Source: CAD feature listing. Evaluate the final solid. Frame: model axes, mm. Face numbers are marked on the shaded views. A direction names the side the tool comes from. Give positions to 0.01 mm unless a question says otherwise; leave off trailing zeros. Order: outer loops, then holes, each group sorted by start corner. A loop starts at its lowest first (then second) coordinate and runs counter-clockwise, first axis right, second up.
from build123d import *

# Parameters (mm, degrees)
MAIN_BODY_DEPTH                 = 75
SKETCH6_W                       = 38
SKETCH6_H                       = 25
BASE_FIT_PLATE_DEPTH            = 4
SKETCH3_W                       = 3.2102875
SKETCH3_H                       = 3
FRONT_SCREW_HOLES_SUPPORT_DEPTH = 6
FRONT_SCREW_HOLES_REACH         = 79.891
SKETCH4_R                       = 1.05
SKETCH7_W                       = 29
SKETCH7_H                       = 20
SKETCH7_R                       = 8
BUTTON_HOLE_DEPTH               = 2
SKETCH8_W                       = 22
SKETCH8_H                       = 25
SKETCH8_W_2                     = 13.3
SKETCH8_H_2                     = 21.3
SWITCH_HOLE_DEPTH               = 8
SKETCH9_R                       = 1.1
BASE_SCREW_HOLES_DEPTH          = 81.051545894


with BuildPart() as part:
    # Sketch1 → Main Body (new body)
    with BuildSketch(Plane(origin=(0, 0, 0), x_dir=(1, 0, 0), z_dir=(0, 1, 0))):
        with BuildLine():
            Line((0, 4.2897125), (-3.715, 2.14485625))
            Line((-3.715, 2.14485625), (-3.715, -2.14485625))
            Line((-3.715, -2.14485625), (0, -4.2897125))
            Line((0, -4.2897125), (0, -7.5))
            ThreePointArc((0, -7.5), (-7.5, 0), (0, 7.5))
            Line((0, 7.5), (0, 4.2897125))
        make_face()
    extrude(amount=MAIN_BODY_DEPTH)

    # Sketch6 → Base Fit Plate (add)
    with BuildSketch(Plane(origin=(-5, 0, 0), x_dir=(0, 0, -1), z_dir=(1, 0, 0))):
        with Locations((0, -2.5)):
            Rectangle(SKETCH6_W, SKETCH6_H)
    extrude(amount=-BASE_FIT_PLATE_DEPTH)

    # Sketch3 → Front Screw Holes Support (add)
    with BuildSketch(Plane(origin=(0, 0, 0), x_dir=(0, 0, -1), z_dir=(1, 0, 0))):
        with Locations((-5.89485625, 1.5)):
            Rectangle(SKETCH3_W, SKETCH3_H)
        with Locations((-5.89485625, 73.5)):
            Rectangle(SKETCH3_W, SKETCH3_H)
    front_screw_holes_support = extrude(amount=-FRONT_SCREW_HOLES_SUPPORT_DEPTH)

    # Sketch4 → Front Screw Holes (cut, up to next)
    with BuildSketch(Plane(origin=(0, 0, 0), x_dir=(0, 0, -1), z_dir=(1, 0, 0)), mode=Mode.PRIVATE) as front_screw_holes_sk1:
        with Locations((-5.89485625, 73.5)):
            Circle(SKETCH4_R)
    front_screw_holes_tool1 = extrude(front_screw_holes_sk1.sketch, amount=-FRONT_SCREW_HOLES_REACH, mode=Mode.PRIVATE) & part.part
    # Sketch4 → Front Screw Holes (cut, up to next)
    with BuildSketch(Plane(origin=(0, 0, 0), x_dir=(0, 0, -1), z_dir=(1, 0, 0)), mode=Mode.PRIVATE) as front_screw_holes_sk2:
        with Locations((-5.89485625, 1.5)):
            Circle(SKETCH4_R)
    front_screw_holes_tool2 = extrude(front_screw_holes_sk2.sketch, amount=-FRONT_SCREW_HOLES_REACH, mode=Mode.PRIVATE) & part.part
    front_screw_holes_1 = front_screw_holes_tool1.solids().sort_by_distance((0, 73.5, 5.894856))[0]
    add(front_screw_holes_1, mode=Mode.SUBTRACT)
    front_screw_holes_2 = front_screw_holes_tool2.solids().sort_by_distance((0, 1.5, 5.894856))[0]
    add(front_screw_holes_2, mode=Mode.SUBTRACT)
    front_screw_holes = front_screw_holes_1 + front_screw_holes_2  # Front Screw Holes as one shape, for the pattern or mirror that repeats it

    # Back Screw Holes and Support: Front Screw Holes Support, Front Screw Holes across plane
    add(front_screw_holes_support.mirror(Plane.XY))
    add(front_screw_holes.mirror(Plane.XY), mode=Mode.SUBTRACT)

    # Sketch7 → Button Hole (add)
    with BuildSketch(Plane(origin=(-5, 0, 0), x_dir=(0, 0, -1), z_dir=(1, 0, 0))):
        with Locations((12, 20)):
            Rectangle(SKETCH7_W, SKETCH7_H)
        with Locations((16, 20)):
            Circle(SKETCH7_R, mode=Mode.SUBTRACT)
    extrude(amount=-BUTTON_HOLE_DEPTH)

    # Sketch8 → Switch Hole (add)
    with BuildSketch(Plane(origin=(-5, 0, 0), x_dir=(0, 0, -1), z_dir=(1, 0, 0))):
        with Locations((15, 42)):
            Rectangle(SKETCH8_W, SKETCH8_H)
        with Locations((15, 42)):
            Rectangle(SKETCH8_W_2, SKETCH8_H_2, mode=Mode.SUBTRACT)
    extrude(amount=-SWITCH_HOLE_DEPTH)

    # Sketch9 → Base Screw Holes (cut, through all)
    with BuildSketch(Plane.ZY.offset(9)):
        with Locations((-13, 3)):
            Circle(SKETCH9_R)
        with Locations((13, 3)):
            Circle(SKETCH9_R)
    extrude(amount=-BASE_SCREW_HOLES_DEPTH, mode=Mode.SUBTRACT)


solid = part.part
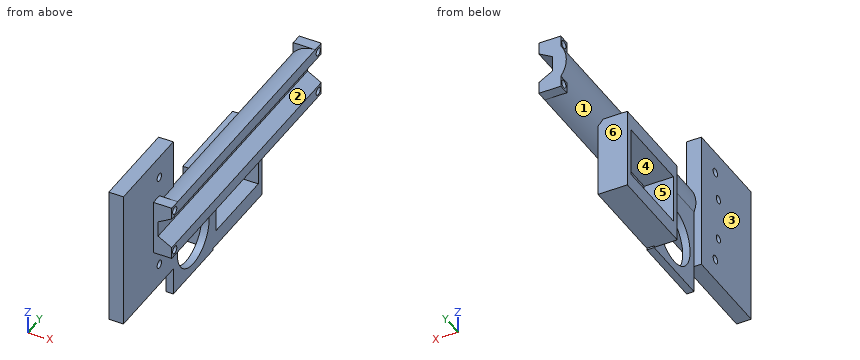
(1) Draft query along Z for the marked faces 5 and 6. Return one class per face: +Z half, -Z half, draft (parallel to the pull), parting line (faces both ways), or undercut.
(2) Section C-C, the plane x = -2.5. Return loops of the section in (y, z), plus the area to 3 significant figures.
(3) Access query for the marked faces 1, 2, 3 and 4. Directions: +Z, -Z, +X, -X, +Y, -Y. A direction counts if a zero-diameter tool reaches every point of the face in a straight line with its end or side. Return the directions, or none.
(4) Pin query (flat end, axial travel): pin 1 Ø4.5 at (x, y) = (-8, 1) entering from -Z; pin 2 Ø1.5 at (y, z) = (74, -5.5) entering from -X; pin 3 Ø4 at (x, z) = (-10, -13.5) entering from +Y. Return the tip coordinate at first contact, or that it passes through.
(5) Section B-B, the plane y = 20. Return loops of the section in (x, z) (3 decimals), plus the area to 3 significant figures.
(6) Line query: line 1 along Y through (x, z) = (-11, -11); line 2 along Y through (x, z) = (-8.5, -7.5); line 3 along Z through (x, y) = (-11.5, 42). Output: solid intervals per line, ascending.
(7) Section D-D, the plane y = 73.5. Return loops of the section in (x, z) (3 decimals).
(8) Section A-A, the plane z = 13. Return loops of the section in (x, y).
Checks:
1. face 5: undercut
1. face 6: draft
2. outline: (0, -7.5) - (3, -7.5) - (3, -7.07) - (72, -7.07) - (72, -7.5) - (75, -7.5) - (75, -2.85) - (0, -2.85) - close; (0, 2.85) - (75, 2.85) - (75, 7.5) - (72, 7.5) - (72, 7.07) - (3, 7.07) - (3, 7.5) - (0, 7.5) - close; hole circle Ø2.1 at (1.5, -5.89); hole circle Ø2.1 at (1.5, 5.89); hole circle Ø2.1 at (73.5, -5.89); hole circle Ø2.1 at (73.5, 5.89)
2. area: 625 mm2
3. face 1: none
3. face 2: +X, +Y, -Y
3. face 3: +Z, -Z, -X, -Y
3. face 4: +X, -X
4. pin 1: stops at z = -19
4. pin 2: stops at x = -6
4. pin 3: stops at y = 54.5
5. outline: (-7, -26.5) - (-5, -26.5) - (-5, -24) - (-7, -24) - close; (-7, -8) - (-5, -8) - (-5, -5.59) arc R7.5 ccw to (0, -7.5) - (0, -4.29) - (-3.715, -2.145) - (-3.715, 2.145) - (0, 4.29) - (0, 7.5) arc R7.5 ccw to (-7, -2.693) - close
5. area: 76.7 mm2
6. line 1: y = 29.5 to 31.35, 52.65 to 54.5
6. line 2: y = -15 to 10, 29.5 to 54.5
6. line 3: z = -26 to -21.65, -8.35 to -4
7. outline: (-6, -7.5) - (0, -7.5) - (0, -6.945) - (-6, -6.945) - close; (-6, -4.845) - (0, -4.845) - (0, -4.29) - (-3.715, -2.145) - (-3.715, 2.145) - (0, 4.29) - (0, 4.845) - (-6, 4.845) - (-6, 4.5) arc R7.5 ccw to (-6, -4.5) - close; (-6, 6.945) - (0, 6.945) - (0, 7.5) - (-6, 7.5) - close
8. outline: (-9, -15) - (-5, -15) - (-5, 1.9) - (-9, 1.9) - close; (-9, 4.1) - (-5, 4.1) - (-5, 10) - (-9, 10) - close
